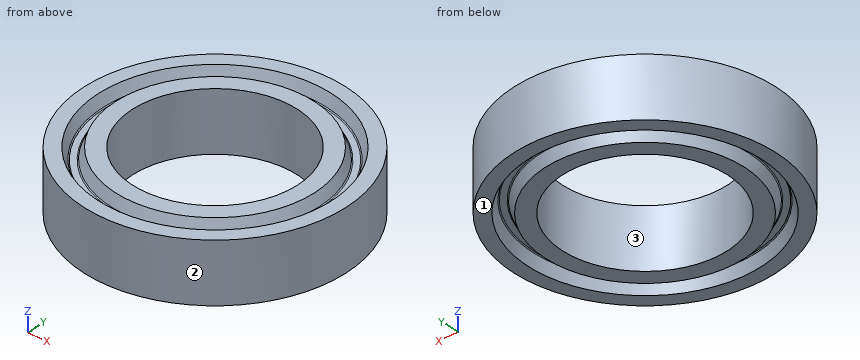
```python
from build123d import *

# Parameters (mm, degrees)
F0_R     = 90.5
F0_R_2   = 57
F1_DEPTH = 41.1


with BuildPart() as f1:
    # F0 (on Top) → F1 (new body)
    with BuildSketch(Plane.XY):
        with Locations((117.5, 0)):
            Circle(F0_R)
        with Locations((117.5, 0)):
            Circle(F0_R_2, mode=Mode.SUBTRACT)
    extrude(amount=F1_DEPTH)

    # F2 (on Front) → F3 (revolve, cut)
    with BuildSketch(Plane.XZ):
        with BuildLine():
            Line((45.685055, 33.667415), (48.84, 41.1))
            Line((48.84, 41.1), (36.93, 41.1))
            Line((36.93, 41.1), (40.084945, 33.667415))
            ThreePointArc((40.084945, 33.667415), (40.379799, 33.312891), (40.821349, 33.18))
            Line((40.821349, 33.18), (44.948651, 33.18))
            ThreePointArc((44.948651, 33.18), (45.390201, 33.312891), (45.685055, 33.667415))
        make_face()
        with BuildLine():
            ThreePointArc((45.685055, 7.432585), (45.390201, 7.787109), (44.948651, 7.92))
            Line((44.948651, 7.92), (40.821349, 7.92))
            ThreePointArc((40.821349, 7.92), (40.379799, 7.787109), (40.084945, 7.432585))
            Line((40.084945, 7.432585), (36.93, 0))
            Line((36.93, 0), (48.84, 0))
            Line((48.84, 0), (45.685055, 7.432585))
        make_face()
    revolve(axis=Axis((117.5, 0, 20.55), (0, 0, -1)), mode=Mode.SUBTRACT)


solid = f1.part
```
Input: part model. Units: mm. Frame: model coordinates. Face numbers are marked on the shaded views. Coordinates: 2 decimals unless noted, no trailing zeros. Order: outer loops, then holes, each group sorted by start corner. A loop starts at its lowest first (then second) coordinate and runs counter-clockwise, first axis right, second up. Notation, with made-up numbers: (82, 48) - (140, 48) arc R20 ccw to (140, 53) - close; hole circle Ø7 at (-19.5, 64.25). An arc over 180 degrees is marked (long way). Return JSON: item names as keys, results as strings.
Q1. Ray query, probe 1 along Y at (x, z) = (117, 16); probe 2 along Y at (x, z) = (180, 7); probe 3 along Y at (x, z) = (132, 37). Return the intervals inside material, ascending.
The answers:
{"probe 1": "y = -90.5 to -57, 57 to 90.5", "probe 2": "y = -65.45 to -45.99, -35 to 35, 45.99 to 65.45", "probe 3": "y = -89.33 to -77.48, -68.89 to -55.12, 55.12 to 68.89, 77.48 to 89.33"}
Q2. Cut plane D-D (z = 11). Return loops of the section in (x, y), then the cut area to 3 significant figures.
The answers:
{"outline": "circle Ø181 at (117.5, 0); hole circle Ø114 at (117.5, 0)", "area": "15,500 mm2"}
Q3. First-contact query: pin 1 (8 mm diameter, centred on x = 184, z = 15.5, fed in from +Y); pin 2 (12 mm diameter, centred on x = 126.5, z = 35, fed in from +Y); pin 3 (4 mm diameter, centred on y = -37, z = 21.5, fed in from +X). Flat tips, straight axial feed; report the tip coordinate or a pass-through.
The answers:
{"pin 1": "stops at y = 65.45", "pin 2": "stops at y = 90.45", "pin 3": "stops at x = 200.96"}
Q4. Draft query along Y for the marked faces 1, 2 and 3. Return one class per face: +Y half, -Y half, draft (parallel to the pull), parting line (faces both ways), or undercut.
The answers:
{"face 1": "draft", "face 2": "parting line", "face 3": "undercut"}
Q5. Cut plane C-C (z = 38). Return loops of the section in (x, y), then the cut area to 3 significant figures.
The answers:
{"outline": "circle Ø181 at (117.5, 0); circle Ø139.95 at (117.5, 0); hole circle Ø158.51 at (117.5, 0); hole circle Ø114 at (117.5, 0)", "area": "11,200 mm2"}
